Could you check a few things on this model? Use its own coordinates, in mm. Face numbers are marked on the shaded views. A direction names the side the tool comes from. Give positions to 0.01 mm unless a question says otherwise; leave off trailing zeros. Write each loop counter-clockwise with the first axis right and the second up, starting at its lowest first coordinate (ties: lowest second). Pieces come first, ordered by that corner, then holes. Notation, with made-up numbers: (73.5, -1) - (113.5, -1) arc R18 ccw to (113.5, 32) - close; hole circle Ø1 at (-8.5, 28). An arc over 180 degrees is marked (long way). Answer in a Markdown table with one row per item.
Autodesk Inventor part; units mm, degrees
ref_plane "YZ Plane" through (0, 0, 0) normal (1, 0, 0) x (0, 1, 0)
ref_plane "XZ Plane" through (0, 0, 0) normal (0, 1, 0) x (-1, 0, 0)
ref_plane "XY Plane" through (0, 0, 0) normal (0, 0, 1) x (1, 0, 0)
sketch "Sketch1" plane through (0, 0, 0) normal (0, 0, 1) x (1, 0, 0)
  line L0 (-9.9228, -20) -> (-13.5328, -20)
  line L1 (-13.5328, -20) -> (-13.5328, -16)
  line L2 (-13.5328, -16) -> (-9.9228, -16)
  line L3 (-9.9228, -16) -> (-9.9228, -20)
  line L4 (-9.9228, -20) -> (-9.9228, -55)
  line L5 (-9.9228, -55) -> (-11.9228, -55)
  line L6 (-11.9228, -55) -> (-11.9228, -20)
  point P0 (0, 0)
  dimension "d0" = 3.61
  dimension "d1" = 4
  dimension "d3" = 2
  dimension "d16" = 35
revolve "Revolution1" add sketch "Sketch1" angle 360 about axis through (-9.9228, -20, 0) along (0, -1, 0)
chamfer "Chamfer1" distance 0.4 angle 45 1 edges at (-6.3128, -16, 0)
sketch "Boceto2" plane through (-9.9228, -16, 0) normal (0, 1, 0) x (1, 0, 0)
  line L0 (1.1641, -1.3443) -> (-0.5821, -1.6803)
  line L1 (-0.5821, -1.6803) -> (-1.7462, -0.336)
  line L2 (-1.7462, -0.336) -> (-1.1641, 1.3443)
  line L3 (-1.1641, 1.3443) -> (0.5821, 1.6803)
  line L4 (0.5821, 1.6803) -> (1.7462, 0.336)
  line L5 (1.7462, 0.336) -> (1.1641, -1.3443)
  point P0 (9.9228, 0)
  point P1 (0, 0)
  dimension "d11" = 3.08
extrude "Extrusión1" cut sketch "Boceto2" against normal blind 2
thread "Rosca1"
properties part number "Tornillo Allen cabeza cilindrica M4x35mm"
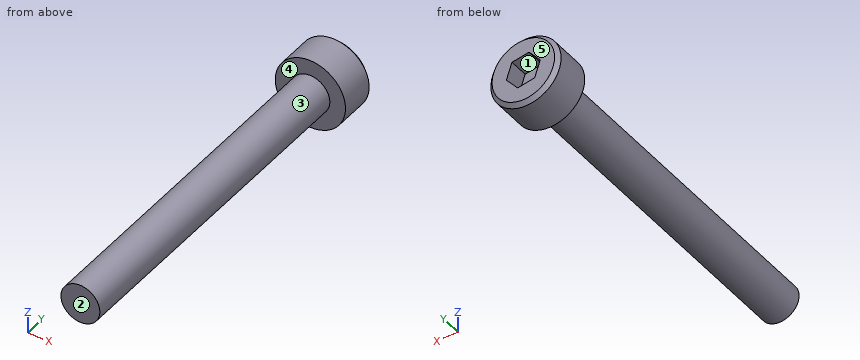
1) Will these pins go through, and if not, where does the flat tip stop? P1, Ø2.5, axis at x = -10, z = -0.5, coming from the +Y side; P2, Ø3, axis at y = -31.5, z = 2.5, coming from the -X side; P3, Ø1.5, axis at x = -8, y = -28.5, coming from the -Z side.
Check values:
| item | result |
|---|---|
| P1 | stops at y = -16 |
| P2 | stops at x = -11.65 |
| P3 | stops at z = -1.62 |
2) If I drill on line 1 (Y direction, x = -7.5, z = 0.5); line 2 (X direction, y = -24, z = 0); line 3 (Y direction, x = -8.25, z = -0.25), over which ranges is the centre line in solid material (lowest first)?
Check values:
| item | result |
|---|---|
| line 1 | y = -20 to -16 |
| line 2 | x = -11.92 to -7.92 |
| line 3 | y = -55 to -18 |
3) We'd pull the mould along Z, two halves only. Please class the marked faces 1, 2 and 3: +Z half, -Z half, draft (parallel to the pull), parting line (faces both ways), or undercut.
Check values:
| item | result |
|---|---|
| face 1 | undercut |
| face 2 | draft |
| face 3 | parting line |
4) Imagine slicing it at A-A (y = -34.5). List the corners of the cut face in (x, z) for me.
Check values:
| item | result |
|---|---|
| outline | circle Ø4 at (-9.92, 0) |
5) On a 3-axis mill with a long thin cutter (end or side, diameter ignored), from which of +Z, -Z, +X, -X, +Y, -Y can I reach the whole of each face in a straight line? I mean the marked faces 4 and 5. Say none if no direction works.
Check values:
| item | result |
|---|---|
| face 4 | -Y |
| face 5 | +Z, -Z, +X, -X, +Y |
6) Imagine slicing it at B-B (z = 0). List the corners of the cut face in (x, y) for me, then the cut area to 3 significant figures.
Check values:
| item | result |
|---|---|
| outline | (-13.53, -20) - (-11.92, -20) - (-11.92, -55) - (-7.92, -55) - (-7.92, -20) - (-6.31, -20) - (-6.31, -16.4) - (-6.71, -16) - (-8.29, -16) - (-8.29, -18) - (-11.55, -18) - (-11.55, -16) - (-13.13, -16) - (-13.53, -16.4) - close |
| area | 162 mm2 |
